Input: dimensioned drawing with shaded views. Units: mm. Origin: part minimum x, y, z. Coordinates: 2 decimals unless noted, no trailing zeros. Order: outer loops, then holes, each group sorted by start corner. A loop starts at its lowest first (then second) coordinate and runs counter-clockwise, first axis right, second up.
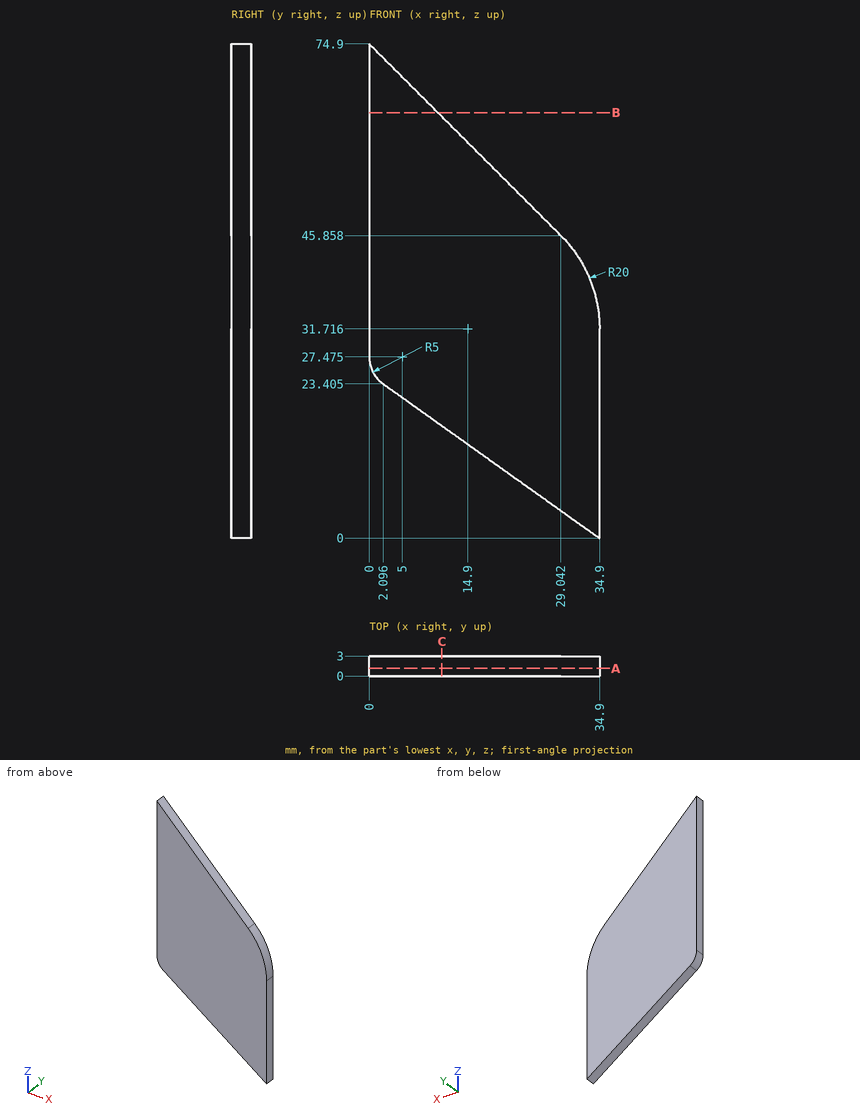
1. Section query C-C on x = 11. Return loops of the section in (y, z).
Findings:
outline: (0, 17.05) - (3, 17.05) - (3, 63.9) - (0, 63.9) - close
2. Ray query, line 1 (X direction, y = 1.05, z = 32); line 2 (X direction, y = 1, z = 37.5) (1 decimal); line 3 (Z direction, x = 1.5, y = 2.9) (1 decimal). Return the intervals inside material, ascending.
Findings:
line 1: x = 0 to 34.9
line 2: x = 0 to 34
line 3: z = 23.9 to 73.4
3. Pin query (flat end, axial travel): P1, Ø1, axis at x = 9, y = 1.5, coming from the -Z side. Return the tip coordinate at first contact, or that it passes through.
Findings:
P1: stops at z = 18.12
4. Section query A-A on y = 1.15. Return loops of the section in (x, z) (1 decimal).
Findings:
outline: (0, 27.5) arc R5 ccw to (2.1, 23.4) - (34.9, 0) - (34.9, 31.7) arc R20 ccw to (29, 45.9) - (0, 74.9) - close
5. Section query B-B on z = 64.5. Return loops of the section in (x, y), plus the area to 3 significant figures.
Findings:
outline: (0, 0) - (10.4, 0) - (10.4, 3) - (0, 3) - close
area: 31.2 mm2
